Job drawing, mm, ordinate dimensions from the low corner. One solid piece. Round coordinates to 2 decimals unless told otherwise and drop trailing zeros. Loops run counter-clockwise (first coordinate to the right, second up) from the corner with the lowest first, then second, coordinate; pieces in that order, holes last.
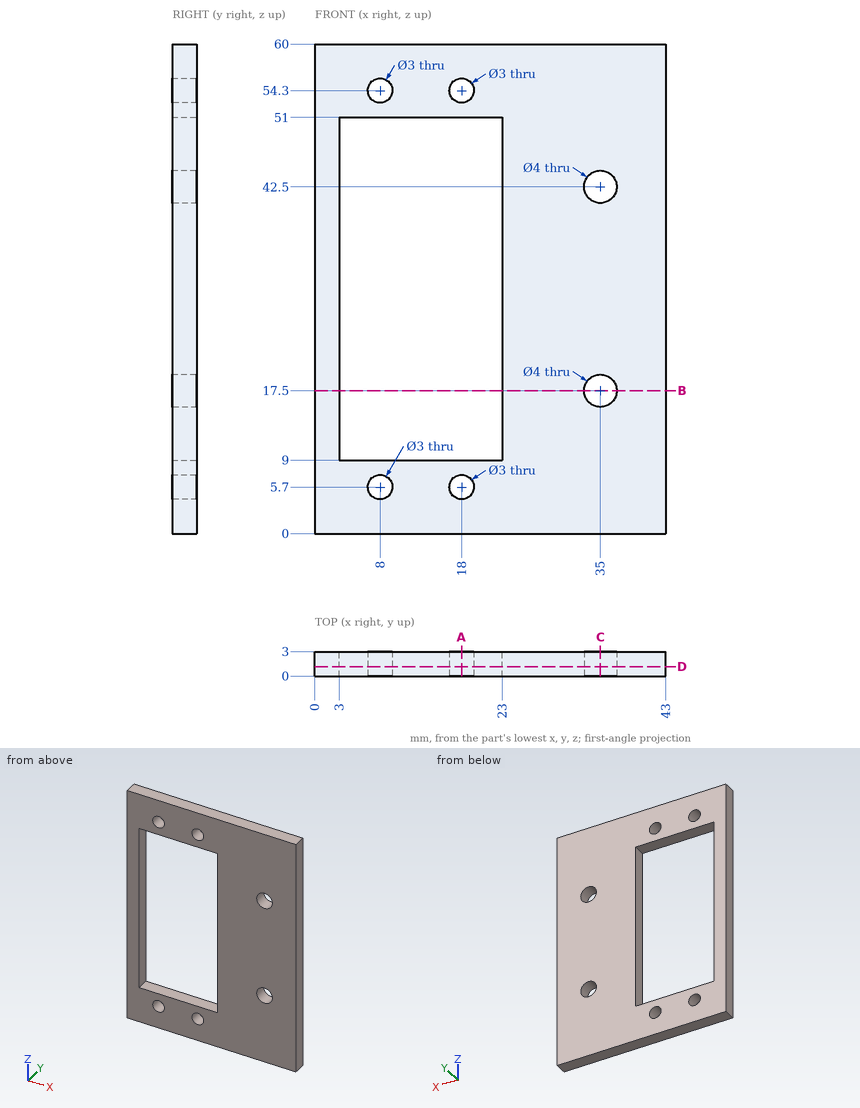
1) Slice it at D-D, the plane y = 1.15. Give the cut face in (x, z), then the cut area to 3 significant figures.
Values:
outline: (0, 0) - (43, 0) - (43, 60) - (0, 60) - close; hole (3, 9) - (23, 9) - (23, 51) - (3, 51) - close; hole circle Ø3 at (8, 5.7); hole circle Ø3 at (8, 54.3); hole circle Ø3 at (18, 5.7); hole circle Ø3 at (18, 54.3); hole circle Ø4 at (35, 17.5); hole circle Ø4 at (35, 42.5)
area: 1,690 mm2
2) Slice it at C-C, the plane x = 35. Give the cut face in (y, z).
Values:
outline: (0, 0) - (3, 0) - (3, 15.5) - (0, 15.5) - close; (0, 19.5) - (3, 19.5) - (3, 40.5) - (0, 40.5) - close; (0, 44.5) - (3, 44.5) - (3, 60) - (0, 60) - close
3) Wall check: line 1 along X through (y, z) = (1.2, 17.5); line 2 along Z through (x, y) = (19, 0.6); line 3 along X through (y, z) = (1.4, 5.7). Give the ranges that are in metal, low to high.
Values:
line 1: x = 0 to 3, 23 to 33, 37 to 43
line 2: z = 0 to 4.58, 6.82 to 9, 51 to 53.18, 55.42 to 60
line 3: x = 0 to 6.5, 9.5 to 16.5, 19.5 to 43
4) Slice it at A-A, the plane x = 18. Give the cut face in (y, z), then the cut area to 3 significant figures.
Values:
outline: (0, 0) - (3, 0) - (3, 4.2) - (0, 4.2) - close; (0, 7.2) - (3, 7.2) - (3, 9) - (0, 9) - close; (0, 51) - (3, 51) - (3, 52.8) - (0, 52.8) - close; (0, 55.8) - (3, 55.8) - (3, 60) - (0, 60) - close
area: 36.0 mm2
5) Slice it at B-B, the plane z = 17.5. Give the cut face in (x, y), then the cut area to 3 significant figures.
Values:
outline: (0, 0) - (3, 0) - (3, 3) - (0, 3) - close; (23, 0) - (33, 0) - (33, 3) - (23, 3) - close; (37, 0) - (43, 0) - (43, 3) - (37, 3) - close
area: 57.0 mm2
6) Drop a flat-ended pin along its axis: pin 1 Ø4 at (x, z) = (8, 5.7) entering from -Y. Give the stop position or say it passes through.
Values:
pin 1: stops at y = 0
